```python
from build123d import *

# Parameters (mm, degrees)
F1_DEPTH = 50
F2_T     = -2


with BuildPart() as f1:
    # F0 (on Front) → F1 (new body)
    with BuildSketch(Plane.XZ):
        with BuildLine():
            ThreePointArc((42, 0), (0, -9.24759), (-42, 0))
            Line((-42, 0), (-42.021068, -25.047362))
            ThreePointArc((-42.021068, -25.047362), (-0.124227, -34.247281), (41.772614, -25.047362))
            Line((41.772614, -25.047362), (42, 0))
        make_face()
    extrude(amount=F1_DEPTH)

    # F2
    f2_openings = [f1.faces().sort_by_distance(p)[0] for p in [
        (0, -25, -9.24759),
    ]]
    offset(amount=F2_T, openings=f2_openings)


solid = f1.part
```
CAD build for the part. Positions are in the model's coordinates, mm. A direction names the side the tool comes from. Round coordinates to 2 decimals unless told otherwise and drop trailing zeros. Write each loop counter-clockwise with the first axis right and the second up, starting at its lowest first coordinate (ties: lowest second). Pieces come first, ordered by that corner, then holes. Notation, with made-up numbers: (12, 32) - (65, 32) arc R24 ccw to (65, 45) - close; hole circle Ø3 at (19, 34). An arc over 180 degrees is marked (long way). Return JSON: item names as keys, results as strings. Group by question number.
Item 1: Mould opens along Y. For faces 3 (the face through (-1, 0, -17)), 4 (the face through (-0.729, -24.65, -34.245)), 5 (the face through (-1, -48, -16)), 6 (the face through (-0.693, -24.678, -32.246)) say: +Y half, -Y half, draft (parallel to the pull), parting line (faces both ways), or undercut.
Item 2: Band-saw the part on B-B on z = -17. List the corners of the cut face in (x, y), plus the area to 3 significant figures.
Item 3: Band-saw the part on A-A on z = -4. List the corners of the cut face in (x, y).
Item 4: Flat gauge pins, fed straight in: pin 1 Ø10 at (y, z) = (-32, -17.5) entering from -X; pin 2 Ø1 at (x, y) = (15.5, -34) entering from +Z; pin 3 Ø6 at (x, y) = (-8, -25.5) entering from +Z. Where does each tip first touch, or does it go through?
Item 5: Band-saw the part on C-C on x = -24. List the corners of the cut face in (y, z).
Item 6: 3-axis set-ups, long thin cutter, end or side, ignore diameter. For faces 1 (the face through (-1, -2, -16)), 2 (the face through (3.41, -48.96, -9.19)): which of +Z, -Z, +X, -X, +Y, -Y reach the whole face in a straight line?
Item 7: Probe probe 1 along Y at (x, z) = (-11, -26.5); probe 2 along X at (y, z) = (-9.5, -9); probe 3 along Z at (x, y) = (-0.5, -3). List the from-to ranges inside material, lowest first.
Item 8: Band-saw the part on D-D on y = -40. List the corners of the cut face in (x, z), plus the area to 3 significant figures.
Resolved:
{
 "1": {"face 3": "+Y half", "face 4": "draft", "face 5": "undercut", "face 6": "undercut"},
 "2": {"outline": "(-42.01, -50) - (41.85, -50) - (41.85, 0) - (-42.01, 0) - close; hole (-40.01, -48) - (39.85, -48) - (39.85, -2) - (-40.01, -2) - close", "area": "519 mm²"},
 "3": {"outline": "(-42, -50) - (-31.97, -50) - (-31.97, -48) - (-40, -48) - (-40, -2) - (-31.97, -2) - (-31.97, 0) - (-42, 0) - close; (31.97, -50) - (41.96, -50) - (41.96, 0) - (31.97, 0) - (31.97, -2) - (39.96, -2) - (39.96, -48) - (31.97, -48) - close"},
 "4": {"pin 1": "stops at x = -42.02", "pin 2": "stops at z = -30.91", "pin 3": "stops at z = -31.64"},
 "5": {"outline": "(-50, -31.36) - (0, -31.36) - (0, -6.32) - (-2, -6.32) - (-2, -29.29) - (-48, -29.29) - (-48, -6.32) - (-50, -6.32) - close"},
 "6": {"face 1": "+Z", "face 2": "+Z, +Y, -Y"},
 "7": {"probe 1": "y = -50 to -48, -2 to 0", "probe 2": "x = -42.01 to -40.01, 39.92 to 41.92", "probe 3": "z = -34.25 to -32.25"},
 "8": {"outline": "(-42.02, -25.05) arc R100 ccw to (41.77, -25.05) - (42, 0) arc R100 cw to (39.99, -0.9) - (39.78, -23.75) arc R98 cw to (-40.02, -23.76) - (-40, -0.9) arc R100 cw to (-42, 0) - close", "area": "264 mm²"}
}
